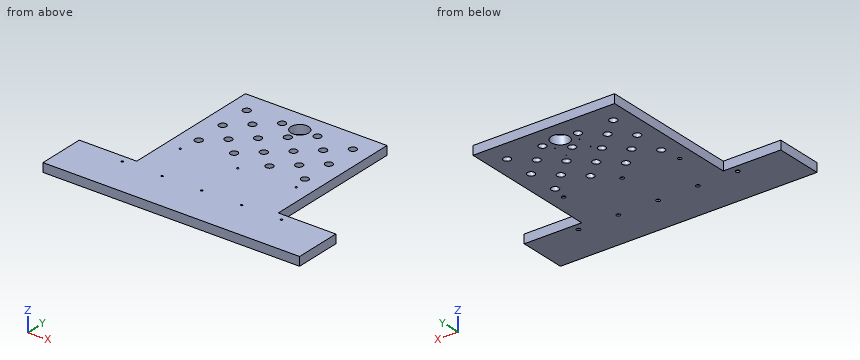
```python
from build123d import *

# Parameters (mm, degrees)
BOSS_EXTRUDE1_DEPTH                            = 19.05
SKETCH2_R                                      = 7.9375
CUT_EXTRUDE1_DEPTH                             = 451.68227514
CSK_FOR_8_FLAT_HEAD_MACHINE_SCREW1_D           = 4.4958
CSK_FOR_8_FLAT_HEAD_MACHINE_SCREW1_CSINK_D     = 8.4328
CSK_FOR_8_FLAT_HEAD_MACHINE_SCREW1_CSINK_ANGLE = 82
HOLE1_D                                        = 38.1
F_5_64_0_07813_DIAMETER_HOLE1_D                = 1.984502
F_5_64_0_07813_DIAMETER_HOLE1_DEPTH            = 11.1252
F_5_64_0_07813_DIAMETER_HOLE1_TIP              = 0.59620455


with BuildPart() as part:
    # Sketch1 → Boss-Extrude1 (new body)
    with BuildSketch(Plane.XY):
        Polygon((-152.4, 50.8), (-152.4, 355.6), (152.4, 355.6), (152.4, 50.8), (276.225, 50.8), (276.225, -50.8), (-276.225, -50.8), (-276.225, 50.8), align=None)
    extrude(amount=BOSS_EXTRUDE1_DEPTH)

    # Sketch2 → Cut-Extrude1 (cut, through all)
    with BuildSketch(Plane.XY.offset(19.05)):
        with Locations((-114.3, 309.5625)):
            Circle(SKETCH2_R)
        with Locations((-38.1, 309.5625)):
            Circle(SKETCH2_R)
        with Locations((38.1, 309.5625)):
            Circle(SKETCH2_R)
        with Locations((114.3, 309.5625)):
            Circle(SKETCH2_R)
        with Locations((-76.2, 275.9075)):
            Circle(SKETCH2_R)
        with Locations((0, 275.9075)):
            Circle(SKETCH2_R)
        with Locations((76.2, 275.9075)):
            Circle(SKETCH2_R)
        with Locations((-114.3, 242.2525)):
            Circle(SKETCH2_R)
        with Locations((-38.1, 242.2525)):
            Circle(SKETCH2_R)
        with Locations((38.1, 242.2525)):
            Circle(SKETCH2_R)
        with Locations((114.3, 242.2525)):
            Circle(SKETCH2_R)
        with Locations((76.2, 208.5975)):
            Circle(SKETCH2_R)
        with Locations((0, 208.5975)):
            Circle(SKETCH2_R)
        with Locations((-76.2, 208.5975)):
            Circle(SKETCH2_R)
        with Locations((-114.3, 174.9425)):
            Circle(SKETCH2_R)
        with Locations((-38.1, 174.9425)):
            Circle(SKETCH2_R)
        with Locations((38.1, 174.9425)):
            Circle(SKETCH2_R)
        with Locations((114.3, 174.9425)):
            Circle(SKETCH2_R)
    extrude(amount=-CUT_EXTRUDE1_DEPTH, mode=Mode.SUBTRACT)

    # CSK for #8 Flat Head Machine Screw1 (through all)
    with Locations(Plane(origin=(0, 0, 0), x_dir=(-1, 0, 0), z_dir=(0, 0, -1))):
        with Locations((-171.45, 34.925), (-85.725, 34.925), (0, 34.925), (171.45, 34.925), (85.725, 34.925), (-120.65, 142.579301206), (0, 135.791261042), (120.65, 131.466801206)):
            CounterSinkHole(CSK_FOR_8_FLAT_HEAD_MACHINE_SCREW1_D / 2, CSK_FOR_8_FLAT_HEAD_MACHINE_SCREW1_CSINK_D / 2, counter_sink_angle=CSK_FOR_8_FLAT_HEAD_MACHINE_SCREW1_CSINK_ANGLE)

    # Hole1 (through all)
    with Locations(Plane.XY.offset(19.05)):
        with Locations((0, 309.5625)):
            Hole(HOLE1_D / 2)

    # 5/64 (0.07813) Diameter Hole1
    with Locations(Plane(origin=(0, 0, 0), x_dir=(-1, 0, 0), z_dir=(0, 0, -1))):
        with Locations((-26.305822693, 290.03907182), (-26.307719853, 258.289071876), (26.30582273, 258.285928054), (26.307719891, 290.035927997)):
            Hole(F_5_64_0_07813_DIAMETER_HOLE1_D / 2, depth=F_5_64_0_07813_DIAMETER_HOLE1_DEPTH)
            with Locations((0, 0, -(F_5_64_0_07813_DIAMETER_HOLE1_DEPTH + F_5_64_0_07813_DIAMETER_HOLE1_TIP / 2))):  # 118° drill point
                Cone(0, F_5_64_0_07813_DIAMETER_HOLE1_D / 2, F_5_64_0_07813_DIAMETER_HOLE1_TIP, mode=Mode.SUBTRACT)


solid = part.part
```
Part model, mm, in its own coordinate system. Coordinates: 2 decimals unless noted, no trailing zeros. Order: outer loops, then holes, each group sorted by start corner. A loop starts at its lowest first (then second) coordinate and runs counter-clockwise, first axis right, second up. Notation, with made-up numbers: (-19, 63.25) - (12, 63.25) arc R15 cw to (12, 81.25) - close; hole circle Ø4 at (-33.75, 45). An arc over 180 degrees is marked (long way). Return JSON: item names as keys, results as strings. Group by question number.
Item 1: Drill centre lines: probe 1 along X at (y, z) = (35.5, 6.5) (3 decimals); probe 2 along Y at (x, z) = (0, 11.75) (1 decimal); probe 3 along Y at (x, z) = (38.1, 4) (3 decimals). Where is each one in solid material? Low to high. Write a range as from..to.
Item 2: Cut at A-A (x = -38.1). List the corners of the cut face in (y, z) (3 decimals).
Item 3: Pin check, flat tips, straight feed: pin 1 (14.5 mm diameter, centred on x = 114.3, y = 174.94, fed in from +Z); pin 2 (3 mm diameter, centred on y = 159, z = 16.5, fed in from +X); pin 3 (1.6 mm diameter, centred on x = 26.31, y = 290.04, fed in from -Z); pin 4 (1.2 mm diameter, centred on x = 26.31, y = 258.29, fed in from -Z). Stop position of each tip, or through.
Item 4: Cut at B-B (y = 91). List the corners of the cut face in (x, z), plus the area to 3 significant figures.
Item 5: Cut at C-C (x = 238.5). List the corners of the cut face in (y, z), plus the area to 3 significant figures.
Check values:
{
 "1": {"probe 1": "x = -276.225..-173.623, -169.277..-87.898, -83.552..-2.173, 2.173..83.552, 87.898..169.277, 173.623..276.225", "probe 2": "y = -50.8..32.7, 37.2..133.5, 138..200.7, 216.5..268, 283.8..290.5, 328.6..355.6", "probe 3": "y = -50.8..167.005, 182.88..234.315, 250.19..301.625, 317.5..355.6"},
 "2": {"outline": "(-50.8, 0) - (167.005, 0) - (167.005, 19.05) - (-50.8, 19.05) - close; (182.88, 0) - (234.315, 0) - (234.315, 19.05) - (182.88, 19.05) - close; (250.19, 0) - (301.625, 0) - (301.625, 19.05) - (250.19, 19.05) - close; (317.5, 0) - (355.6, 0) - (355.6, 19.05) - (317.5, 19.05) - close"},
 "3": {"pin 1": "passes through", "pin 2": "stops at x = 152.4", "pin 3": "stops at z = 11.24", "pin 4": "stops at z = 11.36"},
 "4": {"outline": "(-152.4, 0) - (152.4, 0) - (152.4, 19.05) - (-152.4, 19.05) - close", "area": "5,810 mm2"},
 "5": {"outline": "(-50.8, 0) - (50.8, 0) - (50.8, 19.05) - (-50.8, 19.05) - close", "area": "1,940 mm2"}
}
